Check sheet for the modelled part. Datum: model origin and axes. Units: mm. A direction names the side the tool comes from. Give positions to 0.01 mm unless a question says otherwise; leave off trailing zeros. Order: outer loops, then holes, each group sorted by start corner. A loop starts at its lowest first (then second) coordinate and runs counter-clockwise, first axis right, second up.
from build123d import *

# Parameters (mm, degrees)
SKETCH1_W               = 44.45
SKETCH1_H               = 19.05
BODY_DEPTH              = 2.9972
SKETCH2_W               = 6.35
SKETCH2_H               = 2.9972
TAB_DEPTH               = 2.9972
LPATTERN1_COUNT         = 4
LPATTERN1_PITCH         = 12.7
MIRROR1_COPY_1_SKETCH_W = 6.35
MIRROR1_COPY_1_SKETCH_H = 2.9972
MIRROR1_COPY_1_DEPTH    = 2.9972
MIRROR1_COPY_2_SKETCH_W = 6.35
MIRROR1_COPY_2_SKETCH_H = 2.9972
MIRROR1_COPY_2_DEPTH    = 2.9972
MIRROR1_COPY_3_SKETCH_W = 6.35
MIRROR1_COPY_3_SKETCH_H = 2.9972
MIRROR1_COPY_3_DEPTH    = 2.9972
SKETCH3_W               = 44.45
SKETCH3_H               = 19.05
BOSS_EXTRUDE1_DEPTH     = 10.16
SKETCH4_W               = 5.08
SKETCH4_H               = 19.05
BOSS_EXTRUDE2_DEPTH     = 12.7
CHAMFER1_SIZE           = 5.08


with BuildPart() as part:
    # Sketch1 → Body (new body)
    with BuildSketch(Plane.XY):
        Rectangle(SKETCH1_W, SKETCH1_H)
    extrude(amount=BODY_DEPTH)

    # Sketch2 → Tab (add)
    with BuildSketch(Plane(origin=(0, 9.525, 0), x_dir=(1, 0, 0), z_dir=(0, 1, 0))):
        with Locations((-19.05, -1.4986)):
            Rectangle(SKETCH2_W, SKETCH2_H)
    tab = extrude(amount=TAB_DEPTH)

    # LPattern1: Tab ×4
    with Locations(*[(i * LPATTERN1_PITCH, 0, 0) for i in range(1, LPATTERN1_COUNT)]):
        add(tab)

    # Mirror1: Tab across plane
    add(tab.mirror(Plane.ZX))

    # Mirror1 copy 1 sketch → Mirror1 copy 1 (add)
    with BuildSketch(Plane(origin=(12.7, -9.525, 0), x_dir=(1, 0, 0), z_dir=(0, -1, 0))):
        with Locations((-19.05, 1.4986)):
            Rectangle(MIRROR1_COPY_1_SKETCH_W, MIRROR1_COPY_1_SKETCH_H)
    extrude(amount=MIRROR1_COPY_1_DEPTH)

    # Mirror1 copy 2 sketch → Mirror1 copy 2 (add)
    with BuildSketch(Plane(origin=(25.4, -9.525, 0), x_dir=(1, 0, 0), z_dir=(0, -1, 0))):
        with Locations((-19.05, 1.4986)):
            Rectangle(MIRROR1_COPY_2_SKETCH_W, MIRROR1_COPY_2_SKETCH_H)
    extrude(amount=MIRROR1_COPY_2_DEPTH)

    # Mirror1 copy 3 sketch → Mirror1 copy 3 (add)
    with BuildSketch(Plane(origin=(38.1, -9.525, 0), x_dir=(1, 0, 0), z_dir=(0, -1, 0))):
        with Locations((-19.05, 1.4986)):
            Rectangle(MIRROR1_COPY_3_SKETCH_W, MIRROR1_COPY_3_SKETCH_H)
    extrude(amount=MIRROR1_COPY_3_DEPTH)

    # Sketch3 → Boss-Extrude1 (add)
    with BuildSketch(Plane.XY.offset(2.9972)):
        Rectangle(SKETCH3_W, SKETCH3_H)
    extrude(amount=BOSS_EXTRUDE1_DEPTH)

    # Sketch4 → Boss-Extrude2 (add)
    with BuildSketch(Plane(origin=(22.225, 0, 0), x_dir=(0, 0, -1), z_dir=(1, 0, 0))):
        with Locations((-10.6172, 0)):
            Rectangle(SKETCH4_W, SKETCH4_H)
    extrude(amount=BOSS_EXTRUDE2_DEPTH)

    # Chamfer1
    chamfer1_edges = [part.edges().sort_by_distance(p)[0] for p in [
        (34.925, 0, 13.1572),
    ]]
    chamfer(chamfer1_edges, length=CHAMFER1_SIZE - 0.0001)  # a hair under: the kernel refuses the full size


solid = part.part
1) Section check B-B, the plane z = 1.5. Record the cut outline in (x, y) (3 decimals), then the cut area to 3 significant figures.
Recorded:
outline: (-22.225, -12.522) - (-15.875, -12.522) - (-15.875, -9.525) - (-9.525, -9.525) - (-9.525, -12.522) - (-3.175, -12.522) - (-3.175, -9.525) - (3.175, -9.525) - (3.175, -12.522) - (9.525, -12.522) - (9.525, -9.525) - (15.875, -9.525) - (15.875, -12.522) - (22.225, -12.522) - (22.225, 12.522) - (15.875, 12.522) - (15.875, 9.525) - (9.525, 9.525) - (9.525, 12.522) - (3.175, 12.522) - (3.175, 9.525) - (-3.175, 9.525) - (-3.175, 12.522) - (-9.525, 12.522) - (-9.525, 9.525) - (-15.875, 9.525) - (-15.875, 12.522) - (-22.225, 12.522) - close
area: 999 mm2
2) Draft check along X on faces 1 (the face through (-22.225, 0, 6)), 2 (the face through (-9.525, 11, 2)), 3 (the face through (-19, -12.522, 1)). Enter one of: +X half, -X half, draft (parallel to the pull), parting line (faces both ways), or undercut.
Recorded:
face 1: -X half
face 2: undercut
face 3: draft
3) Section check D-D, the plane x = 8. Record the cut outline in (y, z) (3 decimals), then the cut area to 3 significant figures.
Recorded:
outline: (-12.522, 0) - (12.522, 0) - (12.522, 2.997) - (9.525, 2.997) - (9.525, 13.157) - (-9.525, 13.157) - (-9.525, 2.997) - (-12.522, 2.997) - close
area: 269 mm2
4) Depth check by flat-ended pin: pin 1 Ø1.5 at (y, z) = (-11.5, 1) entering from +X (3 decimals); pin 2 Ø1.5 at (x, z) = (15.5, 4) entering from -Y (3 decimals); pin 3 Ø0.9 at (x, y) = (-5, -11.5) entering from +Z. Enter the tip coordinate at first touch or a pass-through.
Recorded:
pin 1: stops at x = 22.225
pin 2: stops at y = -9.525
pin 3: stops at z = 3
5) Set-up check for faces 4 (the face through (-6, -11, 2.997)), 5 (the face through (15.875, 11, 2)), 6 (the face through (-3.175, -11, 1)): record each of +Z, -Z, +X, -X, +Y, -Y from which the full face is reachable in a straight line by a thin tool's end or side.
Recorded:
face 4: +Z, +X, -X, -Y
face 5: +Z, -Z, +Y
face 6: +Z, -Z, -Y
6) Section check A-A, the plane y = 10.75. Record the cut outline in (x, z) (3 decimals), then the cut area to 3 significant figures.
Recorded:
outline: (-22.225, 0) - (-15.875, 0) - (-15.875, 2.997) - (-22.225, 2.997) - close; (-9.525, 0) - (-3.175, 0) - (-3.175, 2.997) - (-9.525, 2.997) - close; (3.175, 0) - (9.525, 0) - (9.525, 2.997) - (3.175, 2.997) - close; (15.875, 0) - (22.225, 0) - (22.225, 2.997) - (15.875, 2.997) - close
area: 76.1 mm2
7) Material ranges on L1, parallel to Z at x = -6, y = -10.25; L2, parallel to X at y = 8, z = 1.25 (3 decimals); L3, parallel to Y at x = 8, z = 7.5 (3 decimals), recorded low to high.
Recorded:
L1: z = 0 to 3
L2: x = -22.225 to 22.225
L3: y = -9.525 to 9.525
